Geometry: final body of the model. Coordinates: model frame, mm. A direction names the side the tool comes from. Give positions to 0.01 mm unless a question says otherwise; leave off trailing zeros. Write each loop counter-clockwise with the first axis right and the second up, starting at its lowest first coordinate (ties: lowest second). Pieces come first, ordered by that corner, then holes. Notation, with made-up numbers: (12, 41.25) -> (24, 41.25) arc R31 ccw to (24, 75.25) -> close; hole circle Ø6 at (19, 75). An arc over 180 degrees is marked (long way). Answer as a JSON object with one key per item and string values.
Autodesk Inventor part; units mm, degrees
ref_plane "YZ Plane" through (0, 0, 0) normal (1, 0, 0) x (0, 1, 0)
ref_plane "XZ Plane" through (0, 0, 0) normal (0, 1, 0) x (-1, 0, 0)
ref_plane "XY Plane" through (0, 0, 0) normal (0, 0, 1) x (1, 0, 0)
sketch "Boceto1" plane through (0, 0, 0) normal (0, 1, 0) x (-1, 0, 0)
  circle A0 centre (0, 0) radius 11
  dimension "d0" = 22
extrude "Extrusión1" add sketch "Boceto1" along normal blind 4
sketch "Boceto2" plane through (0, 4, 0) normal (0, 1, 0) x (1, 0, 0)
  circle A0 centre (0, 0) radius 8
  circle A1 centre (-8, 0) radius 1.5
  circle A2 centre (0, -8) radius 1.5
  circle A3 centre (8, 0) radius 1.5
  circle A4 centre (0, 8) radius 1.5
  dimension "d3" = 16
  dimension "d4" = 3
  dimension "d7" = 360
extrude "Extrusión2" cut sketch "Boceto2" against normal blind 4 contours A0 A3 | A0 A3 | A4 A0 | A0 A4 | A2 A0 | A0 A2 | A1 A0 | A0 A1
sketch "Boceto3" plane through (0, 4, 0) normal (0, 1, 0) x (1, 0, 0)
  circle A0 centre (0, 0) radius 3.5
  dimension "d11" = 7
extrude "Extrusión3" add sketch "Boceto3" along normal blind 22
properties part number "eje_base"
Q1. Cut plane C-C (z = -8). Return the cut outline in (x, y), and give its area (3 significant figures).
Values:
{"outline": "(-7.55, 0) -> (-1.5, 0) -> (-1.5, 4) -> (-7.55, 4) -> close; (1.5, 0) -> (7.55, 0) -> (7.55, 4) -> (1.5, 4) -> close", "area": "48.4 mm²"}
Q2. Cut plane A-A (z = 0). Return the cut outline in (x, y).
Values:
{"outline": "(-11, 0) -> (-9.5, 0) -> (-9.5, 4) -> (-11, 4) -> close; (-6.5, 0) -> (6.5, 0) -> (6.5, 4) -> (3.5, 4) -> (3.5, 26) -> (-3.5, 26) -> (-3.5, 4) -> (-6.5, 4) -> close; (9.5, 0) -> (11, 0) -> (11, 4) -> (9.5, 4) -> close"}
Q3. Material intervals for L1, parallel to Z at x = 0, y = 3.15; L2, parallel to Y at x = -6, z = -4; L3, parallel to Z at x = 8, y = 2.25, sorted ascending. Write a range as from..to.
Values:
{"L1": "-11..-9.5, -6.5..6.5, 9.5..11", "L2": "0..4", "L3": "-7.55..-1.5, 1.5..7.55"}
Q4. Cut plane B-B (x = 0). Return the cut outline in (y, z), and give its area (3 significant figures).
Values:
{"outline": "(0, -11) -> (4, -11) -> (4, -9.5) -> (0, -9.5) -> close; (0, -6.5) -> (4, -6.5) -> (4, -3.5) -> (26, -3.5) -> (26, 3.5) -> (4, 3.5) -> (4, 6.5) -> (0, 6.5) -> close; (0, 9.5) -> (4, 9.5) -> (4, 11) -> (0, 11) -> close", "area": "218 mm²"}
Q5. First-contact query: P1, Ø3.5, axis at x = 8, z = 0, coming from the +Y side; P2, Ø5, axis at x = -0.5, y = 17.5, coming from the +Z side; P3, Ø10, axis at y = 23, z = -2.5, coming from the -X side. Flat tips, straight axial feed; report the tip coordinate or a pass-through.
Values:
{"P1": "y = 4", "P2": "z = 3.5", "P3": "x = -3.5"}
Q6. Cut plane D-D (x = 9). Return the cut outline in (y, z).
Values:
{"outline": "(0, -6.32) -> (4, -6.32) -> (4, -1.12) -> (0, -1.12) -> close; (0, 1.12) -> (4, 1.12) -> (4, 6.32) -> (0, 6.32) -> close"}
Q7. Set-up query: faces 4 (the flat face through (3, 4, 3)), 5 (the cylindrical face through (6.5, 2.03, -0.07)). Return all of +Z, -Z, +X, -X, +Y, -Y with unobstructed straight access to the full face (end or side cutting, diameter ignored); none if empty.
Values:
{"face 4": "+Y", "face 5": "+Y, -Y"}
Q8. Mould query, pull axis Z, two halves, no side actions, for faces 1 (the flat face through (0, 26, 0)), 2 (the cylindrical face through (2.38, 1.97, 10.74)), 3 (the cylindrical face through (-9.5, 2.03, -0.07)). Classes: pulls with the +Z half, pulls with the -Z half, needs draft (parallel to the pull), parting line crosses it, or undercut.
Values:
{"face 1": "needs draft", "face 2": "parting line crosses it", "face 3": "undercut"}
